Design review of the part built by this model. Coordinates are the model's own, in mm. A direction names the side the tool comes from. Round coordinates to 2 decimals unless told otherwise and drop trailing zeros. Loops run counter-clockwise (first coordinate to the right, second up) from the corner with the lowest first, then second, coordinate; pieces in that order, holes last. Notation, with made-up numbers: M 40,-22.75 L 76,-22.75 A15 ccw 76,-10.75 Z; hole C -33,-25 d10. An arc over 180 degrees is marked long. One line per item, written item: value. Start each with the question number.
Item 1: We need section D-D (y = -1). Write out the cut boundary in (x, z), then the cut area to 3 significant figures.
Item 2: We need section A-A (z = 3.5). Write out the cut boundary in (x, y).
Item 3: Mouldability with a two-part tool opening along Y and no side actions: class faces 4 (the flat face through (-14.43, 8.97, 3.45)), 5 (the cylindrical face through (0, -6, 6)), 6 (the cylindrical face through (0, -14, 3)), 7 (the cylindrical face through (-20.747, 0.121, 3.549)) as released by +Y, released by -Y, zero draft, split by the parting line, or undercut.
Item 4: We need section B-B (y = 10.75). Write out the cut boundary in (x, z), then the cut area to 3 significant figures.
Item 5: We need section C-C (x = -6.5). Write out the cut boundary in (y, z).
Item 6: Clearance check with flat-ended pins moving along their axes: pin 1 (5 mm diameter, centred on x = 18, y = 0, fed in from +Z); pin 2 (2.5 mm diameter, centred on y = 9.5, z = 5, fed in from -X); pin 3 (3 mm diameter, centred on y = -11, z = 2, fed in from -X); pin 4 (1.5 mm diameter, centred on x = 2, z = 7.5, fed in from -Y). State where each tip first meets the part, or that it passes through.
Item 7: For faces 1 (the flat face through (0.75, 10, 6)), 2 (the flat face through (14.68, 8.86, 3.45)), 3 (the flat face through (-11, -7, 7)), list the 3-axis set-ups (+Z, -Z, +X, -X, +Y, -Y) from which the entire face can be reached by the end or side of a thin tool; tool diameter is ignored.
Item 8: For line 1 along X through (y, z) = (0, 9.5); line 2 along Z through (x, y) = (-19, -4); line 3 along X through (y, z) = (7.5, 10.5), list the stretches that pass through material, from the lowest coordinate up.
from build123d import *

# Parameters (mm, degrees)
BOSS_EXTRUDE1_DEPTH = 7
SKETCH2_R           = 12.5
BOSS_EXTRUDE2_DEPTH = 5
SKETCH3_R           = 6
CUT_EXTRUDE1_DEPTH  = 13
SKETCH4_R           = 2.75
CUT_EXTRUDE2_DEPTH  = 8
SKETCH5_W           = 1.5
SKETCH5_H           = 20
CUT_EXTRUDE3_DEPTH  = 13


with BuildPart() as part:
    # Sketch1 → Boss-Extrude1 (new body)
    with BuildSketch(Plane.XY):
        with BuildLine():
            Line((-5.611444446, 12.826211102), (-23.5, 5))
            Line((-23.5, 5), (-23.5, -5))
            Line((-23.5, -5), (-5.611444446, -12.826211102))
            ThreePointArc((-5.611444446, -12.826211102), (0, -14), (5.611444446, -12.826211102))
            Line((5.611444446, -12.826211102), (23.5, -5))
            Line((23.5, -5), (23.5, 5))
            Line((23.5, 5), (5.611444446, 12.826211102))
            ThreePointArc((5.611444446, 12.826211102), (0, 14), (-5.611444446, 12.826211102))
        make_face()
    extrude(amount=BOSS_EXTRUDE1_DEPTH)

    # Sketch2 → Boss-Extrude2 (add)
    with BuildSketch(Plane.XY.offset(7)):
        Circle(SKETCH2_R)
    extrude(amount=BOSS_EXTRUDE2_DEPTH)

    # Sketch3 → Cut-Extrude1 (cut, through all)
    with BuildSketch(Plane.XY.offset(12)):
        Circle(SKETCH3_R)
    extrude(amount=-CUT_EXTRUDE1_DEPTH, mode=Mode.SUBTRACT)

    # Sketch4 → Cut-Extrude2 (cut, through all)
    with BuildSketch(Plane.XY.offset(7)):
        with Locations((-18, 0)):
            Circle(SKETCH4_R)
        with Locations((18, 0)):
            Circle(SKETCH4_R)
    extrude(amount=-CUT_EXTRUDE2_DEPTH, mode=Mode.SUBTRACT)

    # Sketch5 → Cut-Extrude3 (cut, through all)
    with BuildSketch(Plane.XY.offset(12)):
        with Locations((0, 15)):
            Rectangle(SKETCH5_W, SKETCH5_H)
    extrude(amount=-CUT_EXTRUDE3_DEPTH, mode=Mode.SUBTRACT)


solid = part.part
A:
1. outline: M -23.5,0 L -20.56,0 L -20.56,7 L -23.5,7 Z; M -15.44,0 L -5.92,0 L -5.92,12 L -12.46,12 L -12.46,7 L -15.44,7 Z; M 5.92,0 L 15.44,0 L 15.44,7 L 12.46,7 L 12.46,12 L 5.92,12 Z; M 20.56,0 L 23.5,0 L 23.5,7 L 20.56,7 Z
1. area: 240 mm2
2. outline: M -23.5,-5 L -5.61,-12.83 A14 ccw 5.61,-12.83 L 23.5,-5 L 23.5,5 L 5.61,12.83 A14 ccw 0.75,13.98 L 0.75,5.95 A6 cw long -0.75,5.95 L -0.75,13.98 A14 ccw -5.61,12.83 L -23.5,5 Z; hole C -18,0 d5.5; hole C 18,0 d5.5
3. face 4: released by +Y
3. face 5: undercut
3. face 6: released by -Y
3. face 7: undercut
4. outline: M -10.36,0 L -0.75,0 L -0.75,12 L -6.38,12 L -6.38,7 L -10.36,7 Z; M 0.75,0 L 10.36,0 L 10.36,7 L 6.38,7 L 6.38,12 L 0.75,12 Z
4. area: 191 mm2
5. outline: M -12.44,0 L 12.44,0 L 12.44,7 L 10.68,7 L 10.68,12 L -10.68,12 L -10.68,7 L -12.44,7 Z
6. pin 1: through
6. pin 2: x = -16.07
6. pin 3: x = -13.21
6. pin 4: y = -13.93
7. face 1: +Z, -Z, +Y
7. face 2: +Z, -Z, +X, +Y
7. face 3: +Z
8. line 1: -12.5 to -6, 6 to 12.5
8. line 2: 0 to 7
8. line 3: -10 to -0.75, 0.75 to 10
